Can you work these out from the drawing? Everything is in mm from the part's minimum corner. Round coordinates to 2 decimals unless told otherwise and drop trailing zeros. Write each loop counter-clockwise with the first axis right and the second up, starting at its lowest first coordinate (ties: lowest second). Pieces come first, ordered by that corner, then holes.
Q1. I'm going to push a flat-ended pin straight in: pin 1 Ø5 at (x, z) = (33.5, 44) entering from +Y. Where does the tip first touch, or does it pass through?
Q2. If we section it at D-D (z = 53): Please give me the cut outline in (x, y).
Q3. If we section it at A-A (y = 15): Please give me the cut outline in (x, z), plus the area to 3 significant figures.
Q4. If we section it at C-C (y = 28): Please give me the cut outline in (x, z).
Q5. If we section it at B-B (x = 40): Please give me the cut outline in (y, z), plus the area to 3 significant figures.
Q6. Please list where these lines run through material, in increasing order: line 1 along Z through (x, y) = (14, 26.5); line 2 along Y through (x, z) = (40, 15); line 3 along Y through (x, z) = (40, 31).
Q7. We'd pull the mould along Y, two halves only. Please class the marked faces 1, 2 and 3: +Y half, -Y half, draft (parallel to the pull), parting line (faces both ways), or undercut.
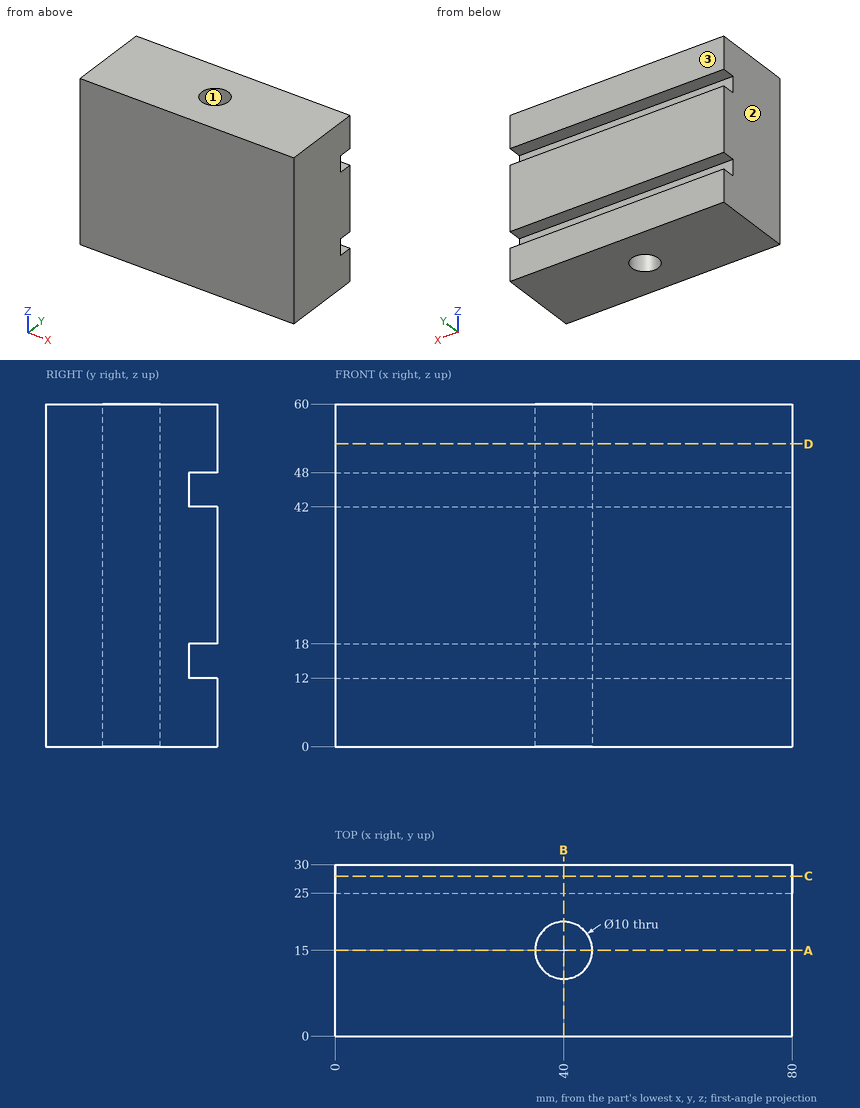
A:
1. pin 1: stops at y = 30
2. outline: (0, 0) - (80, 0) - (80, 30) - (0, 30) - close; hole circle Ø10 at (40, 15)
3. outline: (0, 0) - (35, 0) - (35, 60) - (0, 60) - close; (45, 0) - (80, 0) - (80, 60) - (45, 60) - close
3. area: 4,200 mm2
4. outline: (0, 0) - (80, 0) - (80, 12) - (0, 12) - close; (0, 18) - (80, 18) - (80, 42) - (0, 42) - close; (0, 48) - (80, 48) - (80, 60) - (0, 60) - close
5. outline: (0, 0) - (10, 0) - (10, 60) - (0, 60) - close; (20, 0) - (30, 0) - (30, 12) - (25, 12) - (25, 18) - (30, 18) - (30, 42) - (25, 42) - (25, 48) - (30, 48) - (30, 60) - (20, 60) - close
5. area: 1,140 mm2
6. line 1: z = 0 to 12, 18 to 42, 48 to 60
6. line 2: y = 0 to 10, 20 to 25
6. line 3: y = 0 to 10, 20 to 30
7. face 1: undercut
7. face 2: draft
7. face 3: +Y half
